from build123d import *

# Parameters (mm, degrees)
SKETCH1_R           = 3.5
BOSS_EXTRUDE1_DEPTH = 15
BOSS_EXTRUDE2_DEPTH = 24.9
FILLET1_R           = 3
SKETCH3_R           = 5
BOSS_EXTRUDE3_DEPTH = 100
SKETCH4_R           = 55.5
BOSS_EXTRUDE4_DEPTH = 2.9
CHAMFER1_SIZE       = 2
SKETCH5_R           = 3.4
SKETCH5_R_2         = 2.25
CUT_EXTRUDE1_DEPTH  = 5
CUT_EXTRUDE2_REACH  = 174.423
SKETCH6_R           = 15
SKETCH7_R           = 3.4
CUT_EXTRUDE3_DEPTH  = 6


with BuildPart() as part:
    # Sketch1 → Boss-Extrude1 (new body)
    with BuildSketch(Plane.XY):
        with BuildLine():
            Line((-50, 57), (50, 57))
            ThreePointArc((50, 57), (54.949747468, 54.949747468), (57, 50))
            Line((57, 50), (57, -50))
            ThreePointArc((57, -50), (54.949747468, -54.949747468), (50, -57))
            Line((50, -57), (-50, -57))
            ThreePointArc((-50, -57), (-54.949747468, -54.949747468), (-57, -50))
            Line((-57, -50), (-57, 50))
            ThreePointArc((-57, 50), (-54.949747468, 54.949747468), (-50, 57))
        make_face()
        with Locations((50, 50)):
            Circle(SKETCH1_R, mode=Mode.SUBTRACT)
        with Locations(Location((-50, 50, 0), (0, 0, 180))):
            Circle(SKETCH1_R, mode=Mode.SUBTRACT)
        with Locations(Location((50, -50, 0), (0, 0, 180))):
            Circle(SKETCH1_R, mode=Mode.SUBTRACT)
        with Locations((-50, -50)):
            Circle(SKETCH1_R, mode=Mode.SUBTRACT)
    extrude(amount=BOSS_EXTRUDE1_DEPTH)

    # Sketch2 → Boss-Extrude2 (add)
    with BuildSketch(Plane.XY.offset(15)):
        Polygon((31.388347648, 57), (57, 31.388347648), (57, -31.388347648), (31.388347648, -57), (-31.388347648, -57), (-57, -31.388347648), (-57, 31.388347648), (-31.388347648, 57), align=None)
    extrude(amount=BOSS_EXTRUDE2_DEPTH)

    # Fillet1
    fillet1_edges = [part.edges().sort_by_distance(p)[0] for p in [
        (31.388347648, 57, 27.45),
        (-31.388347648, 57, 27.45),
        (-57, 31.388347648, 27.45),
        (-57, -31.388347648, 27.45),
        (-31.388347648, -57, 27.45),
        (31.388347648, -57, 27.45),
        (57, -31.388347648, 27.45),
        (57, 31.388347648, 27.45),
    ]]
    fillet(fillet1_edges, radius=FILLET1_R)

    # Sketch3 → Boss-Extrude3 (add)
    with BuildSketch(Plane(origin=(57, 0, 0), x_dir=(0, 0, -1), z_dir=(1, 0, 0))):
        with Locations(Location((-6, 20, 0), (0, 0, 270))):
            Circle(SKETCH3_R)
    extrude(amount=BOSS_EXTRUDE3_DEPTH)

    # Sketch4 → Boss-Extrude4 (add)
    with BuildSketch(Plane.XY.offset(39.9)):
        Circle(SKETCH4_R)
    extrude(amount=BOSS_EXTRUDE4_DEPTH)

    # Chamfer1
    chamfer1_edges = [part.edges().sort_by_distance(p)[0] for p in [
        (-55.5, 0, 42.8),
    ]]
    chamfer(chamfer1_edges, length=CHAMFER1_SIZE)

    # Sketch5 → Cut-Extrude1 (cut)
    with BuildSketch(Plane.XY.offset(42.8)):
        with Locations((25, 25)):
            Circle(SKETCH5_R)
        with Locations((0, 38.2)):
            Circle(SKETCH5_R_2)
        with Locations((0, 29.7)):
            Circle(SKETCH5_R_2)
        with Locations((38.2, 0)):
            Circle(SKETCH5_R_2)
        with Locations((29.7, 0)):
            Circle(SKETCH5_R_2)
        with Locations((25, -25)):
            Circle(SKETCH5_R)
        with Locations((0, -38.2)):
            Circle(SKETCH5_R_2)
        with Locations((0, -29.7)):
            Circle(SKETCH5_R_2)
        with Locations((-25, -25)):
            Circle(SKETCH5_R)
        with Locations((-38.2, 0)):
            Circle(SKETCH5_R_2)
        with Locations((-29.7, 0)):
            Circle(SKETCH5_R_2)
        with Locations((-25, 25)):
            Circle(SKETCH5_R)
    extrude(amount=-CUT_EXTRUDE1_DEPTH, mode=Mode.SUBTRACT)

    # Sketch6 → Cut-Extrude2 (cut, up to next)
    with BuildSketch(Plane.XY.offset(42.8), mode=Mode.PRIVATE) as cut_extrude2_sk1:
        Circle(SKETCH6_R)
    cut_extrude2_tool1 = extrude(cut_extrude2_sk1.sketch, amount=-CUT_EXTRUDE2_REACH, mode=Mode.PRIVATE) & part.part
    add(cut_extrude2_tool1.solids().sort_by_distance((0, 0, 42.8))[0], mode=Mode.SUBTRACT)

    # Sketch7 → Cut-Extrude3 (cut)
    with BuildSketch(Plane.XZ.offset(57)):
        with Locations(Location((-25.4, 31.3, 0), (0, 0, 270))):
            Circle(SKETCH7_R)
        with Locations(Location((-25.4, 5.9, 0), (0, 0, 270))):
            Circle(SKETCH7_R)
        with Locations(Location((25.4, 5.9, 0), (0, 0, 90))):
            Circle(SKETCH7_R)
        with Locations(Location((25.4, 31.3, 0), (0, 0, 90))):
            Circle(SKETCH7_R)
    extrude(amount=-CUT_EXTRUDE3_DEPTH, mode=Mode.SUBTRACT)


solid = part.part
Build history of the part. All positions in model axes, mm. A direction names the side the tool comes from. Coordinates: 2 decimals unless noted, no trailing zeros. Write each loop counter-clockwise with the first axis right and the second up, starting at its lowest first coordinate (ties: lowest second). Pieces come first, ordered by that corner, then holes. Notation, with made-up numbers: (-19.5, 36.5) -> (18.5, 36.5) arc R20 ccw to (18.5, 47.5) -> close; hole circle Ø1 at (36, -25). An arc over 180 degrees is marked (long way). Use CSV: the item, a comma, the result in double quotes. Start each with the question number.
Q1. Cut at D-D, the plane z = 6. List the corners of the cut face in (x, y).
Q2. Drill centre lines: probe 1 along Z at (x, y) = (-25, -55); probe 2 along Y at (x, z) = (0, 40.1); probe 3 along X at (y, z) = (-30, 39). Where is each one in solid material? Low to high.
Q3. Flat gauge pins, fed straight in: pin 1 Ø6.5 at (x, y) = (-50, 50) entering from +Z; pin 2 Ø12 at (x, y) = (66, 29.5) entering from +Z; pin 3 Ø3 at (y, z) = (-25, 21.5) entering from +X; pin 4 Ø1.3 at (x, y) = (-29, 0.5) entering from +Z. Where does each tip first touch, or does it go through?
Q4. Cut at A-A, the plane z = 31.3. List the corners of the cut face in (x, y).
Q5. 3-axis set-ups, long thin cutter, end or side, ignore diameter. For faces 1 (the cylindrical face through (106, 25, 6)), 2 (the flat face through (0, -38, 37.8)), 3 (the flat face through (-44.36, 44.03, 27.28)): which of +Z, -Z, +X, -X, +Y, -Y reach the whole face in a straight line?
Q6. Pull direction Z, two halves, no side cores. Call faces 4 (the flat face through (-25, -50, 39.9)), 5 (the flat face through (-25, -51, 31)), 6 (the flat face through (157, 20, 6)): released by +Z, released by -Z, zero draft, split by the parting line, or undercut.
Checked values:
1,outline,"(-57, -50) arc R7 ccw to (-50, -57) -> (-28.8, -57) -> (-28.8, -51) -> (-22, -51) -> (-22, -57) -> (22, -57) -> (22, -51) -> (28.8, -51) -> (28.8, -57) -> (50, -57) arc R7 ccw to (57, -50) -> (57, 15) -> (157, 15) -> (157, 25) -> (57, 25) -> (57, 50) arc R7 ccw to (50, 57) -> (-50, 57) arc R7 ccw to (-57, 50) -> close; hole circle Ø7 at (-50, -50); hole circle Ø7 at (-50, 50); hole circle Ø30 at (0, 0); hole circle Ø7 at (50, -50); hole circle Ø7 at (50, 50)"
2,probe 1,"z = 0 to 2.52, 9.28 to 27.92, 34.68 to 39.9"
2,probe 2,"y = -55.5 to -40.45, -35.95 to -31.95, -27.45 to -15, 15 to 27.45, 31.95 to 35.95, 40.45 to 55.5"
2,probe 3,"x = -57 to -2.23, 2.23 to 57"
3,pin 1,"passes through"
3,pin 2,"stops at z = 9.57"
3,pin 3,"stops at x = 57"
3,pin 4,"stops at z = 37.8"
4,outline,"(-57, -30.15) arc R3 ccw to (-56.12, -32.27) -> (-32.27, -56.12) arc R3 ccw to (-30.15, -57) -> (-28.8, -57) -> (-28.8, -51) -> (-22, -51) -> (-22, -57) -> (22, -57) -> (22, -51) -> (28.8, -51) -> (28.8, -57) -> (30.15, -57) arc R3 ccw to (32.27, -56.12) -> (56.12, -32.27) arc R3 ccw to (57, -30.15) -> (57, 30.15) arc R3 ccw to (56.12, 32.27) -> (32.27, 56.12) arc R3 ccw to (30.15, 57) -> (-30.15, 57) arc R3 ccw to (-32.27, 56.12) -> (-56.12, 32.27) arc R3 ccw to (-57, 30.15) -> close; hole circle Ø30 at (0, 0)"
5,face 1,"+X"
5,face 2,"+Z"
5,face 3,"+Z, -X, +Y"
6,face 4,"released by +Z"
6,face 5,"undercut"
6,face 6,"zero draft"
